Input: part model. Units: mm. Frame: model coordinates. Face numbers are marked on the shaded views. A direction names the side the tool comes from. Give positions to 0.01 mm unless a question says otherwise; leave off trailing zeros. Write each loop counter-clockwise with the first axis right and the second up, starting at its lowest first coordinate (ties: lowest second). Pieces come first, ordered by that corner, then holes. Notation, with made-up numbers: (-8, 35.5) -> (51, 35.5) arc R30 ccw to (51, 59.5) -> close; hole circle Ø4 at (64, -4). An arc over 180 degrees is marked (long way). Return JSON: item names as keys, results as strings. Group by question number.
Item 1: Section D-D, the plane z = 11. Return loops of the section in (x, y), then the cut area to 3 significant figures.
Item 2: Section B-B, the plane x = -12. Return loops of the section in (y, z).
Item 3: Pin query (flat end, axial travel): P1, Ø4.5, axis at x = 12.5, y = -12.5, coming from the -Z side; P2, Ø9, axis at x = -22.5, y = -12.5, coming from the -Z side; P3, Ø4, axis at x = -22.5, y = -12.5, coming from the +Z side. Return the tip coordinate at first contact, or that it passes through.
Item 4: Section C-C, the plane x = -22.5. Count the separate pieces of the cut face and the enclosed holes in it, then the cut area to 3 significant figures.
Item 5: Set-up query: the marked faces 1 and 2. Return all of +Z, -Z, +X, -X, +Y, -Y with unobstructed straight access to the full face (end or side cutting, diameter ignored); none if empty.
Item 6: Line query: line 1 (Y direction, x = 12.5, z = 0.35); line 2 (X direction, y = 12, z = 0); line 3 (Z direction, x = 4.5, y = 1). Output: solid intervals per line, ascending. Write a range as [from, to].
Item 7: Section A-A, the plane y = -35. Return loops of the section in (x, z), then the cut area to 3 significant figures.
Item 8: Mould query, pull axis Y, two halves, no side actions, for the marked faces 3, 4, 5 and 6. Classes: released by +Y, released by -Y, zero draft, split by the parting line, or undercut.
from build123d import *

# Parameters (mm, degrees)
SKETCH1_W               = 60
SKETCH1_H               = 100
BOSS_EXTRUDE1_DEPTH     = 35
CUT_EXTRUDE1_DEPTH      = 86.586213843
CUT_EXTRUDE1_DEPTH_BACK = 86.586213843
SKETCH3_R               = 12
SKETCH3_W               = 16
SKETCH3_H               = 4
CUT_EXTRUDE2_DEPTH      = 86.586213843
CUT_EXTRUDE2_DEPTH_BACK = 86.586213843
SKETCH4_W               = 27.5
SKETCH4_H               = 30
SKETCH5_R               = 1.5
CUT_EXTRUDE3_DEPTH      = 12
SKETCH6_R               = 2.75
CUT_EXTRUDE4_DEPTH      = 2
SKETCH7_W               = 60
SKETCH7_H               = 100
BOSS_EXTRUDE2_DEPTH     = 6
SKETCH11_W              = 3
SKETCH11_H              = 40
CUT_EXTRUDE8_DEPTH      = 50
SKETCH9_R               = 1.5
CUT_EXTRUDE9_DEPTH      = 8
SKETCH12_R              = 2.85
CUT_EXTRUDE10_DEPTH     = 1


with BuildPart() as part:
    # Sketch1 → Boss-Extrude1 (new body)
    with BuildSketch(Plane.XY):
        Rectangle(SKETCH1_W, SKETCH1_H)
    extrude(amount=BOSS_EXTRUDE1_DEPTH)

    # Sketch3 → Cut-Extrude1 (cut, two sides: drawn at the far end of the back side and taken through both)
    with BuildSketch(Plane(origin=(30, 0, 0), x_dir=(0, 0, -1), z_dir=(1, 0, 0)).offset(-CUT_EXTRUDE1_DEPTH_BACK)):
        with Locations((-17.5, 35)):
            Circle(SKETCH3_R)
        with Locations(Location((-17.5, -35, 0), (0, 0, 180))):
            Circle(SKETCH3_R)
        with Locations((-17.5, 16)):
            Rectangle(SKETCH3_W, SKETCH3_H)
    extrude(amount=CUT_EXTRUDE1_DEPTH + CUT_EXTRUDE1_DEPTH_BACK, mode=Mode.SUBTRACT)

    # Sketch4 → Cut-Extrude2 (cut, two sides: drawn at the far end of the back side and taken through both)
    with BuildSketch(Plane(origin=(30, 0, 0), x_dir=(0, 0, -1), z_dir=(1, 0, 0)).offset(-CUT_EXTRUDE2_DEPTH_BACK)):
        with Locations((-21.25, -5)):
            Rectangle(SKETCH4_W, SKETCH4_H)
    extrude(amount=CUT_EXTRUDE2_DEPTH + CUT_EXTRUDE2_DEPTH_BACK, mode=Mode.SUBTRACT)

    # Sketch5 → Cut-Extrude3 (cut)
    with BuildSketch(Plane.XZ.offset(-10)):
        with Locations(Location((-18, 20.569825058, 0), (0, 0, 270))):
            Circle(SKETCH5_R)
        with Locations(Location((-6, 20.569825058, 0), (0, 0, 270))):
            Circle(SKETCH5_R)
        with Locations(Location((6, 20.569825058, 0), (0, 0, 270))):
            Circle(SKETCH5_R)
        with Locations(Location((18, 20.569825058, 0), (0, 0, 270))):
            Circle(SKETCH5_R)
    extrude(amount=-CUT_EXTRUDE3_DEPTH, mode=Mode.SUBTRACT)

    # Sketch6 → Cut-Extrude4 (cut)
    with BuildSketch(Plane.XZ.offset(-10)):
        with Locations(Location((-18, 20.569825058, 0), (0, 0, 270))):
            Circle(SKETCH6_R)
        with Locations(Location((-6, 20.569825058, 0), (0, 0, 270))):
            Circle(SKETCH6_R)
        with Locations(Location((6, 20.569825058, 0), (0, 0, 270))):
            Circle(SKETCH6_R)
        with Locations(Location((18, 20.569825058, 0), (0, 0, 270))):
            Circle(SKETCH6_R)
    extrude(amount=-CUT_EXTRUDE4_DEPTH, mode=Mode.SUBTRACT)

    # Sketch7 → Boss-Extrude2 (add)
    with BuildSketch(Plane(origin=(0, 0, 0), x_dir=(-1, 0, 0), z_dir=(0, 0, -1))):
        Rectangle(SKETCH7_W, SKETCH7_H)
    extrude(amount=BOSS_EXTRUDE2_DEPTH)

    # Sketch11 → Cut-Extrude8 (cut)
    with BuildSketch(Plane.ZY.offset(30)):
        with Locations((-3, 0)):
            Rectangle(SKETCH11_W, SKETCH11_H)
    extrude(amount=-CUT_EXTRUDE8_DEPTH, mode=Mode.SUBTRACT)

    # Sketch9 → Cut-Extrude9 (cut)
    with BuildSketch(Plane(origin=(0, 0, -6), x_dir=(-1, 0, 0), z_dir=(0, 0, -1))):
        with Locations((-12.5, 12.5)):
            Circle(SKETCH9_R)
        with Locations(Location((-12.5, -12.5, 0), (0, 0, 180))):
            Circle(SKETCH9_R)
        with Locations((22.5, -12.5)):
            Circle(SKETCH9_R)
        with Locations(Location((22.5, 12.5, 0), (0, 0, 180))):
            Circle(SKETCH9_R)
    extrude(amount=-CUT_EXTRUDE9_DEPTH, mode=Mode.SUBTRACT)

    # Sketch12 → Cut-Extrude10 (cut)
    with BuildSketch(Plane(origin=(0, 0, -6), x_dir=(-1, 0, 0), z_dir=(0, 0, -1))):
        with Locations((-12.5, 12.5)):
            Circle(SKETCH12_R)
        with Locations((22.5, 12.5)):
            Circle(SKETCH12_R)
        with Locations((22.5, -12.5)):
            Circle(SKETCH12_R)
        with Locations((-12.5, -12.5)):
            Circle(SKETCH12_R)
    extrude(amount=-CUT_EXTRUDE10_DEPTH, mode=Mode.SUBTRACT)


solid = part.part
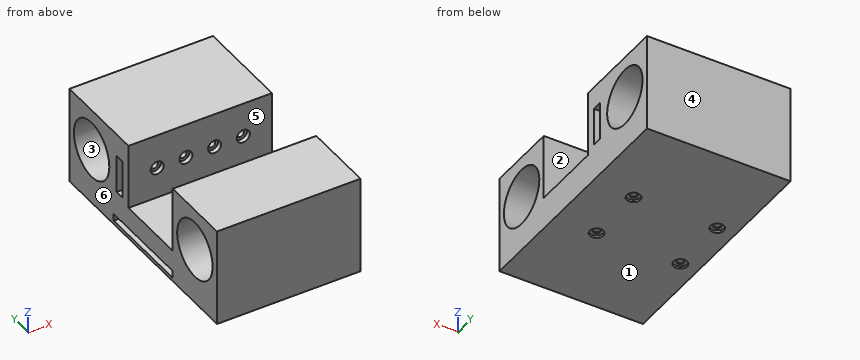
Answer below:
{
 "1": {"outline": "(-30, -50) -> (30, -50) -> (30, -45.09) -> (-30, -45.09) -> close; (-30, -24.91) -> (30, -24.91) -> (30, -20) -> (-30, -20) -> close; (-30, 10) -> (30, 10) -> (30, 14) -> (-30, 14) -> close; (-30, 18) -> (30, 18) -> (30, 24.91) -> (-30, 24.91) -> close; (-30, 45.09) -> (30, 45.09) -> (30, 50) -> (-30, 50) -> close", "area": "1,540 mm2"},
 "2": {"outline": "(-50, -6) -> (50, -6) -> (50, 35) -> (10, 35) -> (10, 7.5) -> (-20, 7.5) -> (-20, 35) -> (-50, 35) -> close; hole circle Ø24 at (-35, 17.5); hole (-20, -4.5) -> (20, -4.5) -> (20, -1.5) -> (-20, -1.5) -> close; hole (14, 9.5) -> (18, 9.5) -> (18, 25.5) -> (14, 25.5) -> close; hole circle Ø24 at (35, 17.5)"},
 "3": {"P1": "stops at z = -5", "P2": "stops at z = -6", "P3": "stops at z = 7.5"},
 "4": {"separate pieces": "2", "enclosed holes": "3", "area": "2,150 mm2"},
 "5": {"face 1": "-Z, +X, -X, +Y, -Y", "face 2": "+Z, +X, -X"},
 "6": {"line 1": "y = [-50, -14], [-11, 11], [14, 50]", "line 2": "x = [-30, -23.91], [-21.09, 11.09], [13.91, 30]", "line 3": "z = [-6, -4.5], [-1.5, 7.5]"},
 "7": {"outline": "(-30, -6) -> (30, -6) -> (30, 5.5) -> (-30, 5.5) -> close; (-30, 29.5) -> (30, 29.5) -> (30, 35) -> (-30, 35) -> close", "area": "1,020 mm2"},
 "8": {"face 3": "undercut", "face 4": "released by +Y", "face 5": "undercut", "face 6": "zero draft"}
}
